```python
from build123d import *

# Parameters (mm, degrees)
F0_W           = 110
F0_H           = 30
F1_DEPTH       = 12.5
F3_D           = 5.5
F3_DEPTH       = 12
F3_TIP         = 1.6523667023
F5_DEPTH       = 25
F7_D           = 6.5
F10_DEPTH      = 3
F10_DEPTH_BACK = 20.0010001
F11_W          = 5.2
F11_H          = 8.5
F12_DEPTH      = 20
F13_R          = 10


# Not quite as in the source:
# - a pattern or mirror of a feature is missing from the dataset's text; its kind, count and spacing are read off the source's solid


with BuildPart() as f1:
    # F0 (on Right) → F1 (new body, symmetric)
    with BuildSketch(Plane.YZ):
        with Locations((0, 15)):
            Rectangle(F0_W, F0_H)
    extrude(amount=F1_DEPTH, both=True)

    # F3
    with Locations(Plane.YZ.offset(12.5)):
        with Locations((-45, 15), (45, 15)):
            Hole(F3_D / 2, depth=F3_DEPTH)
            with Locations((0, 0, -(F3_DEPTH + F3_TIP / 2))):  # 118° drill point
                Cone(0, F3_D / 2, F3_TIP, mode=Mode.SUBTRACT)

    # F4 (on face) → F5 (cut, through all)
    with BuildSketch(Plane.YZ.offset(12.5)):
        with BuildLine():
            Line((-35, 0), (35, 0))
            ThreePointArc((35, 0), (0, 20), (-35, 0))
        make_face()
    extrude(amount=-F5_DEPTH, mode=Mode.SUBTRACT)

    # F7 (through all)
    with Locations(Plane.XY.offset(30)):
        with Locations((-4.5, 17.5), (-4.5, -17.5)):
            Hole(F7_D / 2)

    # F9 (on offset) → F10 (cut, two sides)
    with BuildSketch(Plane.XY.offset(20)) as f10_sk:
        Polygon((-9.75, -20.5310889132), (-4.5, -23.5621778265), (0.75, -20.5310889132), (0.75, -14.4689110868), (-4.5, -11.4378221735), (-9.75, -14.4689110868), align=None)
    f10 = extrude(amount=F10_DEPTH, mode=Mode.SUBTRACT) + extrude(f10_sk.sketch, amount=-F10_DEPTH_BACK, mode=Mode.SUBTRACT)

    # F10_copies: F10 across plane
    add(f10.mirror(Plane.ZX), mode=Mode.SUBTRACT)

    # F11 (on face) → F12 (cut)
    with BuildSketch(Plane.XY.offset(30)):
        with Locations((5.9, -45)):
            Rectangle(F11_W, F11_H)
    f12 = extrude(amount=-F12_DEPTH, mode=Mode.SUBTRACT)

    # F12_copies: F12 across plane
    add(f12.mirror(Plane.ZX), mode=Mode.SUBTRACT)

    # F13
    f13_edges = [f1.edges().sort_by_distance(p)[0] for p in [
        (-12.5, -55, 15),
        (-12.5, 55, 15),
    ]]
    fillet(f13_edges, radius=F13_R)


solid = f1.part
```
Input: part model. Units: mm. Frame: model coordinates. A direction names the side the tool comes from. Give positions to 0.01 mm unless a question says otherwise; leave off trailing zeros. Write each loop counter-clockwise with the first axis right and the second up, starting at its lowest first coordinate (ties: lowest second). Pieces come first, ordered by that corner, then holes. Notation, with made-up numbers: (50.25, 17.25) - (74.25, 17.25) arc R13 ccw to (74.25, 33.25) - close; hole circle Ø2 at (35.25, -3). An arc over 180 degrees is marked (long way). Write item = value, one per line. Start each with the question number.
1. Section query D-D, the plane y = 30. Output: boundary loops of the cut face in (x, z), then the cut area to 3 significant figures.
2. Mould query, pull axis X, two halves, no side actions, for faces 4 (the flat face through (12.5, -1, 22)), 5 (the flat face through (6, -49.25, 20)), 6 (the flat face through (5, 55, 15)). Classes: released by +X, released by -X, zero draft, split by the parting line, or undercut.
3. Section query B-B, the plane z = 21. Output: boundary loops of the cut face in (x, y), then the cut area to 3 significant figures.
4. Section query C-C, the plane y = -17.5. Output: boundary loops of the cut face in (x, z), then the cut area to 3 significant figures.
5. Section query A-A, the plane z = 4.5. Output: boundary loops of the cut face in (x, y), then the cut area to 3 significant figures.
6. Ray query, L1, parallel to Y at x = 6, z = 24.5; L2, parallel to Z at x = 2.75, y = 45; L3, parallel to Y at x = -4.5, z = 26.25. Return the intervals inside material, ascending.
7. First-contact query: pin 1 Ø2.5 at (y, z) = (-44, 15.5) entering from +X; pin 2 Ø11.5 at (x, y) = (-5.5, 17) entering from -Z; pin 3 Ø3.5 at (y, z) = (45, 15) entering from +X. Flat tips, straight axial feed; report the tip coordinate or a pass-through.
8. Access query for faces 1 (the cylindrical face through (-6.25, 20.24, 26.45)), 2 (the flat face through (6, -40.75, 20)), 3 (the flat face through (0.75, 18, 20)). Directions: +Z, -Z, +X, -X, +Y, -Y. A direction counts if a zero-diameter tool reaches every point of the face in a straight line with its end or side. Return the directions, or none.
Check sheet entries:
q1.outline = (-12.5, 6.77) - (12.5, 6.77) - (12.5, 30) - (-12.5, 30) - close
q1.area = 581 mm2
q2.face_4 = released by +X
q2.face_5 = undercut
q2.face_6 = zero draft
q3.outline = (-12.5, -45) arc R10 ccw to (-2.5, -55) - (12.5, -55) - (12.5, 55) - (-2.5, 55) arc R10 ccw to (-12.5, 45) - close; hole (-9.75, -20.53) - (-4.5, -23.56) - (0.75, -20.53) - (0.75, -14.47) - (-4.5, -11.44) - (-9.75, -14.47) - close; hole (-9.75, 14.47) - (-4.5, 11.44) - (0.75, 14.47) - (0.75, 20.53) - (-4.5, 23.56) - (-9.75, 20.53) - close; hole (3.3, -49.25) - (8.5, -49.25) - (8.5, -40.75) - (3.3, -40.75) - close; hole (3.3, 40.75) - (8.5, 40.75) - (8.5, 49.25) - (3.3, 49.25) - close
q3.area = 2,430 mm2
q4.outline = (-12.5, 16.04) - (-9.75, 16.04) - (-9.75, 23) - (-7.75, 23) - (-7.75, 30) - (-12.5, 30) - close; (-1.25, 23) - (0.75, 23) - (0.75, 16.04) - (12.5, 16.04) - (12.5, 30) - (-1.25, 30) - close
q4.area = 230 mm2
q5.outline = (-12.5, -45) arc R10 ccw to (-2.5, -55) - (12.5, -55) - (12.5, -31.92) - (-12.5, -31.92) - close; (-12.5, 31.92) - (12.5, 31.92) - (12.5, 55) - (-2.5, 55) arc R10 ccw to (-12.5, 45) - close
q5.area = 1,110 mm2
q6.L1 = -55 to -49.25, -40.75 to 40.75, 49.25 to 55
q6.L2 = 0 to 12.25, 17.75 to 30
q6.L3 = -54.8 to -20.75, -14.25 to 14.25, 20.75 to 54.8
q7.pin_1 = 0.27
q7.pin_2 = 13.04
q7.pin_3 = -0.1
q8.face_1 = +Z, -Z
q8.face_2 = +Z
q8.face_3 = -Z
